Autodesk Fusion 360 part; units mm, degrees
sketch "スケッチ1" plane through (0, 0, 0) normal (0, 1, 0) x (1, 0, 0)
  arc A0 (181.8653, -105) -> (181.8653, 105) centre (0, 0) ccw
  line L0 (181.8653, 105) -> (0, 0)
  line L1 (0, 0) -> (181.8653, -105)
  line L2 (0, 0) -> (210, 0)
  arc A1 (168.0089, -97) -> (168.0089, 97) centre (0, 0) ccw
  line L3 (191.3426, 32) -> (135, 32)
  line L4 (135, 32) -> (135, 18)
  line L5 (135, 18) -> (193.1631, 18)
  arc A2 (165, 28.1) -> (165, 21.9) centre (165, 25) ccw
  line L6 (165, 28.1) -> (196, 28.1)
  line L7 (196, 28.1) -> (196, 21.9)
  line L8 (196, 21.9) -> (165, 21.9)
  arc A3 (143, 28.1) -> (143, 21.9) centre (143, 25) ccw
  arc A4 (153, 21.9) -> (153, 28.1) centre (153, 25) ccw
  line L9 (143, 28.1) -> (153, 28.1)
  line L10 (153, 21.9) -> (143, 21.9)
  line L11 (10, 0) -> (184.3138, 100.6401)
  arc A5 (154.1525, -89) -> (154.1525, 89) centre (0, 0) ccw
  line L12 (10, 0) -> (184.3138, -100.6401)
  line L13 (193.1631, -18) -> (167, -18)
  line L14 (163, -32) -> (191.3426, -32)
  arc A6 (133, -11.9) -> (133, -18.1) centre (133, -15) ccw
  arc A7 (143, -18.1) -> (143, -11.9) centre (143, -15) ccw
  arc A8 (165, -21.9) -> (165, -28.1) centre (165, -25) ccw
  line L15 (165, -21.9) -> (196, -21.9)
  line L16 (196, -21.9) -> (196, -28.1)
  line L17 (196, -28.1) -> (165, -28.1)
  line L18 (133, -11.9) -> (143, -11.9)
  line L19 (143, -18.1) -> (133, -18.1)
  arc A9 (183.0742, -85.3689) -> (183.0742, 85.3689) centre (0, 0) ccw
  line L20 (0, 0) -> (183.0742, 85.3689)
  line L21 (0, 0) -> (183.0742, -85.3689)
  line L22 (180, 18) -> (180, -18)
  line L23 (175.1, 32) -> (182.0632, 67)
  line L24 (175.1, -32) -> (182.0632, -67)
  line L25 (167, -18) -> (147, -8)
  line L26 (147, -8) -> (125, -8)
  line L27 (125, -8) -> (125, -22)
  line L28 (125, -22) -> (143, -22)
  line L29 (143, -22) -> (163, -32)
  point P0 (135, 25)
  point P1 (202, 0)
  point P2 (125, -15)
  dimension "d1" = 210
  dimension "d2" = 30
  dimension "d3" = 30
  dimension "d4" = 194
  dimension "d5" = 14
  dimension "d6" = 3.1
  dimension "d7" = 3.1
  dimension "d8" = 10
  dimension "d9" = 8
  dimension "d10" = 31
  dimension "d11" = 12
  dimension "d12" = 25
  dimension "d13" = 135
  dimension "d14" = 30
  dimension "d15" = 10
  dimension "d16" = 178
  dimension "d17" = 30
  dimension "d19" = 3.1
  dimension "d20" = 3.1
  dimension "d23" = 202
  dimension "d24" = 25
  dimension "d25" = 25
  dimension "d29" = 180
  dimension "d34" = 25
  dimension "d35" = 15
  dimension "d36" = 7
  dimension "d37" = 7
  dimension "d38" = 22
  dimension "d39" = 10
  dimension "d40" = 8
  dimension "d41" = 22
  dimension "d42" = 20
  dimension "d43" = 18
  dimension "d44" = 20
  dimension "d45" = 14
  dimension "d46" = 35
  dimension "d47" = 35
extrude "押し出し1" add sketch "スケッチ1" along normal blind 5 contours A0 L2 A1 L12 A9 L21 | A0 L2 A1 L11 A9 L20 | L2 A1 L15 L16 L17 A9 L21 | L2 A1 L6 L7 L8 A9 L20 | L2 A1 L13 L22 | L2 A1 L5 L22 | A1 L14 L24 | A1 A5 L13 L15 | A1 L5 L8 A5 | A1 A5 L14 L17 | A5 L13 L14 A8 L15 L17 L25 L26 L27 L28 L29 | A1 L3 L23 | L3 L4 L5 A2 L6 L8 A5 | A1 L3 L6 A5
hole "穴1" at (183.0742, 0, 85.3689) at (202, 0, 0) at (183.0742, 0, -85.3689) direction (0, 1, 0) diameter 3.2 end through all
fillet "フィレット1" radius 1 10 edges at (184.3138, 2.5, 100.6401) (184.3138, 2.5, -100.6401) (180, 2.5, -18) (180, 2.5, 18) (175.1, 2.5, 32) (175.1, 2.5, -32) (182.0632, 2.5, -67) (182.0632, 2.5, 67) (143, 2.5, 22) (167, 2.5, 18)
fillet "フィレット2" radius 7 4 edges at (135, 2.5, -18) (135, 2.5, -32) (125, 2.5, 8) (125, 2.5, 22)
Geometry: final body of the model. Coordinates: model frame, mm. A direction names the side the tool comes from. Give positions to 0.01 mm unless a question says otherwise; leave off trailing zeros. Write each loop counter-clockwise with the first axis right and the second up, starting at its lowest first coordinate (ties: lowest second). Pieces come first, ordered by that corner, then holes.
1. Section query A-A, the plane x = 159.5. Return loops of the section in (y, z).
2. Draft query along Z for faces 4 (the flat face through (183, 5, 7)), 5 (the cylindrical face through (137.1, 2.5, -30)), 6 (the flat face through (138, 2, 18.1)), 7 (the cylindrical face through (209.995, 2.465, -1.455)). Return one class per face: released by +Z, released by -Z, zero draft, split by the parting line, or undercut.
3. Section query C-C, the plane y = 2.7. Count the separate pieces of the cut face and the enclosed holes in it, then the cut area to 3 significant figures.
4. Section query B-B, the plane z = 25. Return loops of the section in (x, y), then the cut area to 3 significant figures.
5. Reachability of faces 1 (the cylindrical face through (176.746, 2.465, 79.981)), 2 (the flat face through (183, 0, 7)), 3 (the flat face through (180, 2, -28.1)) from +Z, -Z, +X, -X, +Y, -Y: full face, straight path, thin tool, end or side. Return the list, or none.
6. Line query: probe 1 along Z at (x, y) = (170, 3.2); probe 2 along Z at (x, y) = (162.5, 3.9); probe 3 along X at (y, z) = (0.35, 17.5). Output: solid intervals per line, ascending.
7. Pin query (flat end, axial travel): P1, Ø2.5, axis at x = 137, y = 3, coming from the +Z side; P2, Ø1.5, axis at y = 2.5, z = -7, coming from the -X side; P3, Ø2.5, axis at x = 166.5, y = 2, coming from the +Z side. Return the tip coordinate at first contact, or that it passes through.
Computed:
1. outline: (0, -32) - (5, -32) - (5, -18) - (0, -18) - close; (0, 14.25) - (5, 14.25) - (5, 30.25) - (0, 30.25) - close
2. face 4: zero draft
2. face 5: released by -Z
2. face 6: undercut
2. face 7: split by the parting line
3. separate pieces: 1
3. enclosed holes: 7
3. area: 5,450 mm2
4. outline: (149, 0) - (161.9, 0) - (161.9, 5) - (149, 5) - close; (196, 0) - (208.51, 0) - (208.51, 5) - (196, 5) - close
4. area: 127 mm2
5. face 1: -X, +Y, -Y
5. face 2: +Z, -Z, +X, -X, -Y
5. face 3: +Y, -Y
6. probe 1: z = -32 to -28.1, -21.9 to -18, 18 to 21.9, 28.1 to 32
6. probe 2: z = -32 to -26.83, -23.17 to -18, 15.75 to 23.17, 26.83 to 31.75
6. probe 3: x = 125.46 to 131.17, 144.83 to 166, 179.87 to 209.27
7. P1: stops at z = 22
7. P2: stops at x = 180
7. P3: stops at z = 32
